Here's the drawing with two shaded views (mm, measured from the low corner). I have some questions. A direction names the side the tool comes from. Coordinates: 2 decimals unless noted, no trailing zeros. Loops run counter-clockwise (first coordinate to the right, second up) from the corner with the lowest first, then second, coordinate; pieces in that order, holes last.
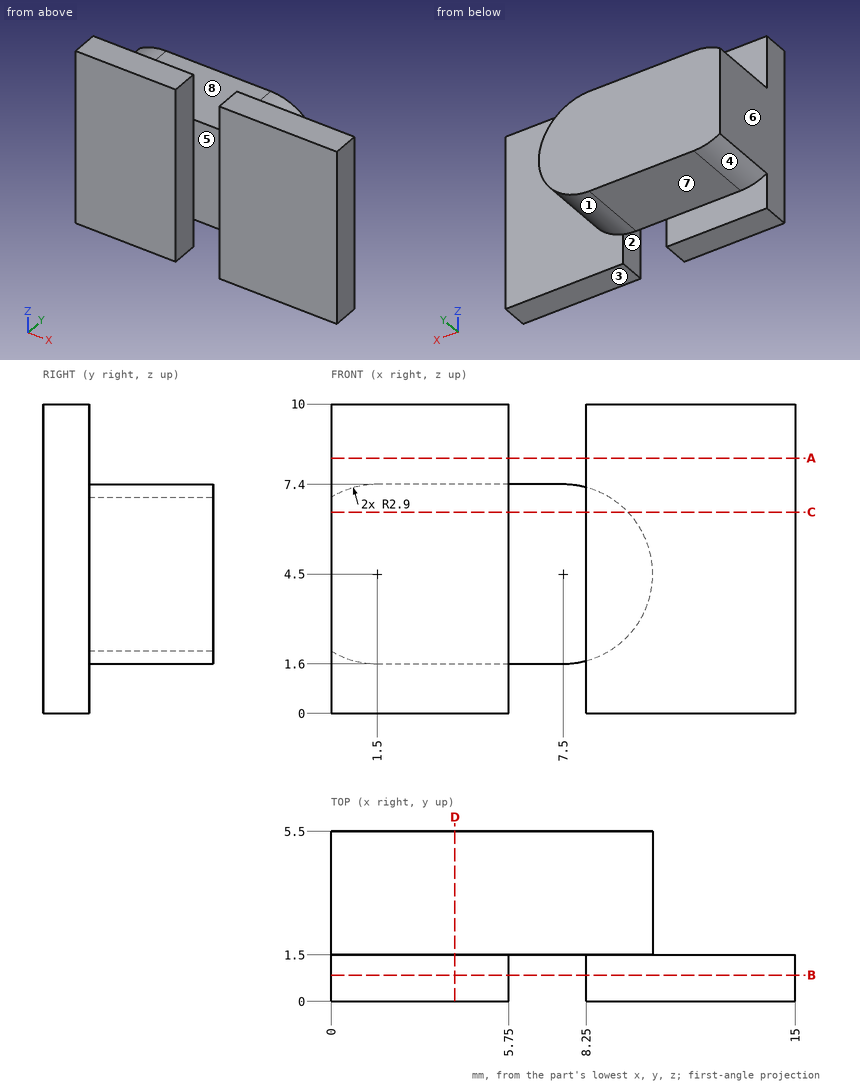
Q1. Suppose I cut it at D-D on x = 4. Write out the boundary of the cut face in (y, z).
Q2. Will these pins go through, and if not, where does the flat tip stop? P1, Ø0.6, axis at x = 2.5, z = 0.5, coming from the +Y side; P2, Ø1.2, axis at x = 3, y = 4.5, coming from the -Z side.
Q3. For the marked faces 4, 5, 6, 7 and 8, which set-ups out of +Z, -Z, +X, -X, +Y, -Y let a thin tool reach every point of the face, with its end or its side?
Q4. Please list where these lines run through material, in increasing order: probe 1 along X at (y, z) = (1.15, 8.25); probe 2 along Z at (x, y) = (5, 3.4); probe 3 along Y at (x, z) = (11.25, 1.5).
Q5. Suppose I cut it at A-A on z = 8.25. Write out the boundary of the cut face in (x, y).
Q6. We'd pull the mould along X, two halves only. Please class the marked faces 1, 2 and 3: pulls with the +X half, pulls with the -X half, needs draft (parallel to the pull), parting line crosses it, or undercut.
Q7. Suppose I cut it at B-B on y = 0.85. Write out the boundary of the cut face in (x, z), and give its area (3 significant figures).
Q8. Suppose I cut it at C-C on z = 6.5. Write out the boundary of the cut face in (x, y), and give its area (4 significant figures).
Check values:
1. outline: (0, 0) - (1.5, 0) - (1.5, 1.6) - (5.5, 1.6) - (5.5, 7.4) - (1.5, 7.4) - (1.5, 10) - (0, 10) - close
2. P1: stops at y = 1.5
2. P2: stops at z = 1.6
3. face 4: -Z, -X, +Y
3. face 5: +Z, -Z, -Y
3. face 6: +Z, -Z, -X, +Y, -Y
3. face 7: -Z, +X, -X, +Y
3. face 8: +Z, +X, -X, +Y
4. probe 1: x = 0 to 5.75, 8.25 to 15
4. probe 2: z = 1.6 to 7.4
4. probe 3: y = 0 to 1.5
5. outline: (0, 0) - (5.75, 0) - (5.75, 1.5) - (0, 1.5) - close; (8.25, 0) - (15, 0) - (15, 1.5) - (8.25, 1.5) - close
6. face 1: pulls with the +X half
6. face 2: undercut
6. face 3: needs draft
7. outline: (0, 0) - (5.75, 0) - (5.75, 10) - (0, 10) - close; (8.25, 0) - (15, 0) - (15, 10) - (8.25, 10) - close
7. area: 125 mm2
8. outline: (0, 0) - (5.75, 0) - (5.75, 1.5) - (8.25, 1.5) - (8.25, 0) - (15, 0) - (15, 1.5) - (9.6, 1.5) - (9.6, 5.5) - (0, 5.5) - close
8. area: 57.15 mm2
